Autodesk Inventor part; units mm, degrees
ref_plane "Work Plane2" through (27.2811, 2.682, 0.7251) normal (1, 0, 0) x (0, 1, 0)
ref_plane "YZ Plane" through (0, 0, 0) normal (1, 0, 0) x (0, 1, 0)
ref_plane "XZ Plane" through (0, 0, 0) normal (0, 1, 0) x (-1, 0, 0)
ref_plane "Work Plane1" through (0, 0, 0) normal (0, 0, 1) x (1, 0, 0)
sketch "Sketch1" plane through (0, 0, 0) normal (0, 0, 1) x (1, 0, 0)
  circle A0 centre (2.6061, 6.2821) radius 1.5 construction
  circle A1 centre (22.6061, 6.2821) radius 1.5 construction
  line L0 (-2.6427, 15.6321) -> (-2.6427, -2.7179) construction
  line L1 (-2.6427, -2.7179) -> (30.1061, -2.7179) construction
  line L2 (30.1061, -2.7179) -> (30.1061, -39.6443) construction
  line L3 (30.1061, -39.6443) -> (66.9651, 7.5331) construction
  line L4 (66.9651, 7.5331) -> (66.9651, 15.6321) construction
  line L5 (66.9651, 15.6321) -> (-2.6427, 15.6321) construction
  circle A2 centre (12.3511, 11.6321) radius 1.45 construction
  circle A3 centre (41.9344, -5.4679) radius 1.45 construction
  circle A4 centre (34.1061, -5.4679) radius 1.45 construction
  circle A5 centre (54.6178, 11.6321) radius 1.45 construction
  circle A6 centre (-0.6427, 11.6823) radius 1.45 construction
  circle A7 centre (29.5857, 11.6321) radius 1.45 construction
  circle A8 centre (51.7579, -5.4342) radius 1.45 construction
  circle A9 centre (34.1061, -24.4536) radius 1.45 construction
  circle A10 centre (47.169, 11.6321) radius 1.45 construction
  line L6 (-7.0605, -146.6377) -> (1.2368, -137.4227) construction
  line L7 (-28.8718, -126.9987) -> (-20.5745, -117.7837) construction
  line L8 (32.1612, -8.9378) -> (42.8353, -8.9378)
  line L9 (42.8353, -8.9378) -> (51.0915, -0.6816)
  line L10 (51.0915, -0.6816) -> (51.0915, 15.6321)
  line L11 (32.1612, -8.9378) -> (32.1612, 15.6321)
  line L12 (32.1612, 15.6321) -> (51.0915, 15.6321)
  circle A11 centre (34.1061, -5.4679) radius 1.55
  circle A12 centre (41.9344, -5.4679) radius 1.55
  circle A13 centre (47.169, 11.6321) radius 1.55
  line L13 (32.1612, 15.6321) -> (51.0915, 15.6321)
  line L14 (51.0915, 15.6321) -> (51.0915, 20.6321)
  line L15 (51.0915, 20.6321) -> (32.1612, 20.6321)
  line L16 (32.1612, 20.6321) -> (32.1612, 15.6321)
  point P0 (0, 0)
  dimension "d0" = 135
  dimension "d1" = 3.1
  dimension "d2" = 3.1
  dimension "d3" = 3.1
  dimension "d16" = 5
extrude "Extrusion1" add sketch "Sketch1" along normal blind 4
sketch "Sketch2" plane through (32.1612, -8.9378, 0) normal (-1, 0, 0) x (0, 0, 1)
  line L0 (0, 0) -> (0, 29.5699)
  line L1 (0, 0) -> (4, 0)
  line L2 (4, 29.5699) -> (4, 0)
  line L3 (10.8285, 6.8285) -> (15.2199, 11.2199)
  line L4 (15.2199, 11.2199) -> (28.65, 11.2199)
  line L5 (28.65, 11.2199) -> (28.65, 29.5699)
  line L6 (28.65, 29.5699) -> (0, 29.5699)
  line L7 (10.8285, 6.8285) -> (0, 6.8285)
  line L8 (0, 0) -> (0, 8.2562)
  line L9 (0, 29.5699) -> (4, 29.5699)
  ellipse E0 centre (24.65, -131.1602) end of major axis (23.05, -131.1602) minor radius 1.189
  ellipse E1 centre (4.65, -131.1602) end of major axis (3.05, -131.1602) minor radius 1.189
  point P0 (0, 8.9378)
  point P1 (0, 6.2199)
  dimension "d8" = 45
ref_plane "Work Plane2" through (27.2811, 2.682, 0.7251) normal (1, 0, 0) x (0, 1, 0)
extrude "Extrusion2" add sketch "Sketch2" along normal up to surface (4.8801 mm away) contours L0 L7 L2 L1 | L0 L6 L2 L7 | L2 L6 L5 L4 L3 L7
sketch "Sketch3" plane through (51.0915, -0.6816, 0) normal (1, 0, 0) x (0, 0, -1)
  circle A0 centre (-24.65, 13.9637) radius 1.5
  circle A1 centre (-4.65, 13.9637) radius 1.5
  ellipse E0 centre (-4.65, -139.4164) end of major axis (-3.05, -139.4164) minor radius 1.189
  ellipse E1 centre (-24.65, -139.4164) end of major axis (-23.05, -139.4164) minor radius 1.189
  point P0 (0, 0.6816)
  dimension "d17" = 3
  dimension "d18" = 3
extrude "Extrusion3" cut sketch "Sketch3" against normal through all
sketch "Sketch4" plane through (51.0915, -0.6816, 0) normal (1, 0, 0) x (0, 0, -1)
  arc A0 (-4, 5.5016) -> (-4, 8.4257) centre (-4.65, 6.9637) ccw
  circle A1 centre (-4.65, 6.9637) radius 3.25
  arc A2 (-4, 12.6118) -> (-4, 15.3155) centre (-4.65, 13.9637) ccw
  circle A3 centre (-4.65, 13.9637) radius 3.2592
  point P0 (0, 0.6816)
  dimension "d13" = 6.5
extrude "Extrusion4" cut sketch "Sketch4" against normal up to surface (18.9303 mm away)
properties part number "cellSTORM_alviumadapter"
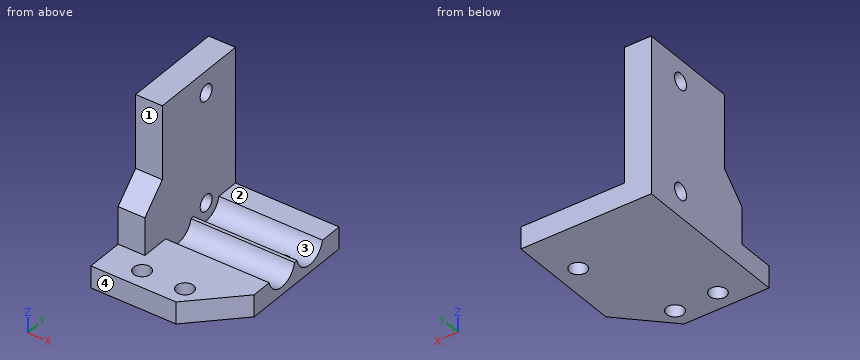
Here's how the part is built. I have some questions about the finished solid (model axes, mm). Face numbers are marked on the shaded views. A direction names the side the tool comes from. Give positions to 0.01 mm unless a question says otherwise; leave off trailing zeros. Write each loop counter-clockwise with the first axis right and the second up, starting at its lowest first coordinate (ties: lowest second). Pieces come first, ordered by that corner, then holes. Notation, with made-up numbers: (-17.5, 57.25) -> (22.5, 57.25) arc R34 cw to (22.5, 94.25) -> close; hole circle Ø6 at (12.25, 20). An arc over 180 degrees is marked (long way). Use one line per item in the form item = value.
1) On a 3-axis mill with a long thin cutter (end or side, diameter ignored), from which of +Z, -Z, +X, -X, +Y, -Y can I reach the whole of each face in a straight line? I mean the marked faces 1, 2, 3 and 4. Say none if no direction works.
Verdict:
face_1 = +Z, +X, -X, -Y
face_2 = +Z, +X, +Y, -Y
face_3 = +Z, +X
face_4 = +Z, -Z, +X, -X, -Y
2) Suppose I cut it at D-D (z = 4.65). Please give me the cut outline in (x, y).
Verdict:
outline = (27.28, -2.11) -> (32.16, -2.11) -> (32.16, 11.78) -> (27.28, 11.78) -> close; (27.28, 14.78) -> (32.16, 14.78) -> (32.16, 20.63) -> (27.28, 20.63) -> close
3) Suppose I cut it at C-C (x = 47.75). Please give me the cut outline in (y, z).
Verdict:
outline = (-4.02, 0) -> (10.2, 0) -> (10.2, 3.6) arc R3.26 cw to (10.09, 4) -> (9.47, 4) arc R3.25 cw to (3.1, 4) -> (-4.02, 4) -> close; (13.07, 0) -> (20.63, 0) -> (20.63, 4) -> (16.48, 4) arc R3.26 cw to (13.07, 1.4) -> close
4) If I drill on L1, parallel to Y at x = 28.7, z = 24.65; L2, parallel to Y at x = 37, z = 2.5; L3, parallel to Y at x = 33.25, z = 3.25, over which ranges is the centre line in solid material (lowest first)? Write a range as [from, to].
Verdict:
L1 = [2.28, 11.78], [14.78, 20.63]
L2 = [-8.94, 3.84], [8.72, 10.83], [15.73, 20.63]
L3 = [-8.94, -6.76], [-4.18, 3.35], [9.22, 10.34], [16.23, 20.63]
5) I'm going to push flat-ended pins straight in: pin 1 (4.5 mm diameter, centred on x = 44, y = 19, fed in from +Z); pin 2 (4 mm diameter, centred on x = 29.5, z = 8.5, fed in from -Y); pin 3 (1.5 mm diameter, centred on x = 30.5, z = 19, fed in from -Y). Where does each tip first touch, or does it pass through?
Verdict:
pin_1 = 4
pin_2 = -2.11
pin_3 = 2.28
6) Suppose I cut it at B-B (y = 14). Please give me the cut outline in (x, z).
Verdict:
outline = (27.28, 0) -> (51.09, 0) -> (51.09, 1.47) -> (32.16, 1.47) -> (32.16, 3.33) -> (27.28, 3.33) -> close; (27.28, 5.97) -> (32.16, 5.97) -> (32.16, 23.33) -> (27.28, 23.33) -> close; (27.28, 25.97) -> (32.16, 25.97) -> (32.16, 28.65) -> (27.28, 28.65) -> close
7) Suppose I cut it at A-A (z = 24.65). Please give me the cut outline in (x, y), and give its area (3 significant figures).
Verdict:
outline = (27.28, 2.28) -> (32.16, 2.28) -> (32.16, 11.78) -> (27.28, 11.78) -> close; (27.28, 14.78) -> (32.16, 14.78) -> (32.16, 20.63) -> (27.28, 20.63) -> close
area = 74.9 mm2
